Can you work these out from the model? Positions are in its coordinate system, mm. A direction names the side the tool comes from. Coordinates: 2 decimals unless noted, no trailing zeros. Order: outer loops, then holes, each group sorted by start corner. A loop starts at its lowest first (then second) coordinate and runs counter-clockwise, first axis right, second up. Notation, with made-up numbers: (75, 27.25) -> (127, 27.25) arc R29 cw to (127, 50.25) -> close; hole circle Ø7 at (40.25, 6.5). An arc over 180 degrees is marked (long way). Return JSON: item names as keys, results as strings. Group by question number.
1) If we section it at A-A, the plane y = 377.75: Please give me the cut outline in (x, z).
2) If I drill on probe 1 along Y at (x, z) = (16, 0); probe 2 along Y at (x, z) = (-7, 8.5); probe 3 along Z at (x, y) = (-1.5, 12.5), over which ranges is the centre line in solid material (lowest first)? Write a range as from..to.
3) If we section it at C-C, the plane y = 18: Please give me the cut outline in (x, z), then the cut area to 3 significant figures.
4) For faces 1 (the cylindrical face through (-1.846, 381.299, -16.888)), 2 (the flat face through (0, -7.009, 0)), 3 (the flat face through (-1.4, 0, -9.3)), which set-ups out of +Z, -Z, +X, -X, +Y, -Y let a thin tool reach every point of the face, with its end or its side?
5) If we section it at B-B, the plane x = 0: Please give me the cut outline in (y, z).
6) Thinking about a two-plate mould opening in X: for faces 4 (the flat face through (-10, -19, 0)), 5 (the flat face through (0, 378, -25)), 6 (the cylindrical face through (-1.846, 381.299, 17.112)), 7 (the flat face through (18, -15, 0)), which applies, +X half, -X half, draft (parallel to the pull), parting line (faces both ways), or undercut?
7) For pin 1 (15 mm diameter, centred on x = 4, y = -15.5, fed in from -Z); pin 2 (4 mm diameter, centred on y = 90, z = -8, fed in from -X); pin 3 (6 mm diameter, centred on x = -4.5, y = 167.5, fed in from +Z); pin 4 (3 mm diameter, centred on y = -22, z = 0, fed in from -X), each with a flat end and sliding along its axis, tell me the tip position at first contact or that it passes through.
from build123d import *

# Parameters (mm, degrees)
SKETCH1_W           = 33
SKETCH1_H           = 18
BOSS_EXTRUDE1_DEPTH = 388
SKETCH3_R           = 4
BOSS_EXTRUDE2_DEPTH = 25
SKETCH4_W           = 36
SKETCH4_H           = 21
BOSS_EXTRUDE3_DEPTH = 30
SKETCH5_W           = 20
SKETCH5_H           = 45.982478268
CUT_EXTRUDE1_DEPTH  = 391.036216267
SKETCH6_R           = 2.5
CUT_EXTRUDE2_DEPTH  = 391.467668316


with BuildPart() as part:
    # Sketch1 → Boss-Extrude1 (new body)
    with BuildSketch(Plane(origin=(0, 0, 0), x_dir=(1, 0, 0), z_dir=(0, 1, 0))):
        Rectangle(SKETCH1_W, SKETCH1_H)
    extrude(amount=BOSS_EXTRUDE1_DEPTH)

    # Sketch3 → Boss-Extrude2 (add, symmetric)
    with BuildSketch(Plane.XY):
        with Locations(Location((0, 377.75, 0), (0, 0, 180))):
            Circle(SKETCH3_R)
    extrude(amount=BOSS_EXTRUDE2_DEPTH, both=True)

    # Sketch4 → Boss-Extrude3 (add)
    with BuildSketch(Plane.XZ):
        Rectangle(SKETCH4_W, SKETCH4_H)
    extrude(amount=BOSS_EXTRUDE3_DEPTH)

    # Sketch5 → Cut-Extrude1 (cut, through all)
    with BuildSketch(Plane.XY.offset(10.5)):
        with Locations((0, -30)):
            Rectangle(SKETCH5_W, SKETCH5_H)
    extrude(amount=-CUT_EXTRUDE1_DEPTH, mode=Mode.SUBTRACT)

    # Sketch6 → Cut-Extrude2 (cut, through all)
    with BuildSketch(Plane(origin=(18, 0, 0), x_dir=(0, 0, -1), z_dir=(1, 0, 0))):
        with Locations((0, -22)):
            Circle(SKETCH6_R)
    extrude(amount=-CUT_EXTRUDE2_DEPTH, mode=Mode.SUBTRACT)


solid = part.part
Result sheet:
{
 "1": {"outline": "(-16.5, -9) -> (-4, -9) -> (-4, -25) -> (4, -25) -> (4, -9) -> (16.5, -9) -> (16.5, 9) -> (4, 9) -> (4, 25) -> (-4, 25) -> (-4, 9) -> (-16.5, 9) -> close"},
 "2": {"probe 1": "y = -30..-24.5, -19.5..388", "probe 2": "y = -7.01..388", "probe 3": "z = -9..9"},
 "3": {"outline": "(-16.5, -9) -> (16.5, -9) -> (16.5, 9) -> (-16.5, 9) -> close", "area": "594 mm2"},
 "4": {"face 1": "-Z", "face 2": "+Z, -Z, -Y", "face 3": "none"},
 "5": {"outline": "(-7.01, -10.5) -> (0, -10.5) -> (0, -9) -> (373.75, -9) -> (373.75, -25) -> (381.75, -25) -> (381.75, -9) -> (388, -9) -> (388, 9) -> (381.75, 9) -> (381.75, 25) -> (373.75, 25) -> (373.75, 9) -> (0, 9) -> (0, 10.5) -> (-7.01, 10.5) -> close"},
 "6": {"face 4": "undercut", "face 5": "draft", "face 6": "parting line", "face 7": "+X half"},
 "7": {"pin 1": "stops at z = -10.5", "pin 2": "stops at x = -16.5", "pin 3": "stops at z = 9", "pin 4": "passes through"}
}
